Job drawing, mm, ordinate dimensions from the low corner. One solid piece. Round coordinates to 2 decimals unless told otherwise and drop trailing zeros. Write each loop counter-clockwise with the first axis right and the second up, starting at its lowest first coordinate (ties: lowest second). Pieces come first, ordered by that corner, then holes.
1) Flat gauge pins, fed straight in: pin 1 (3 mm diameter, centred on x = 4, y = 32, fed in from +Z) (1 decimal); pin 2 (4 mm diameter, centred on x = 19.5, y = 27, fed in from +Z) (1 decimal); pin 3 (2 mm diameter, centred on x = 18, y = 56.5, fed in from -Z) (1 decimal); pin 4 (2 mm diameter, centred on y = 33, z = 21, fed in from +X). Where does each tip first touch, or does it go through?
2) Pull direction X, two halves, no side cores. Call the marked faces 1 and 2: +X half, -X half, draft (parallel to the pull), parting line (faces both ways), or undercut.
3) Saw through at C-C (y = 38.5). Write the cut outline in (x, z) (1 decimal).
4) Saw through at A-A (x = 20.5). Write the cut outline in (y, z) (1 decimal).
5) Saw through at B-B (z = 27.5). Write the cut outline in (x, y) (1 decimal).
6) Wall check: probe 1 along X at (y, z) = (24, 31); probe 2 along Y at (x, z) = (19.75, 4.5) (1 decimal); probe 3 along Z at (x, y) = (21, 10) (1 decimal). Give the ranges that are in metal, low to high.
7) Saw through at D-D (x = 17.5). Write the cut outline in (y, z) (1 decimal).
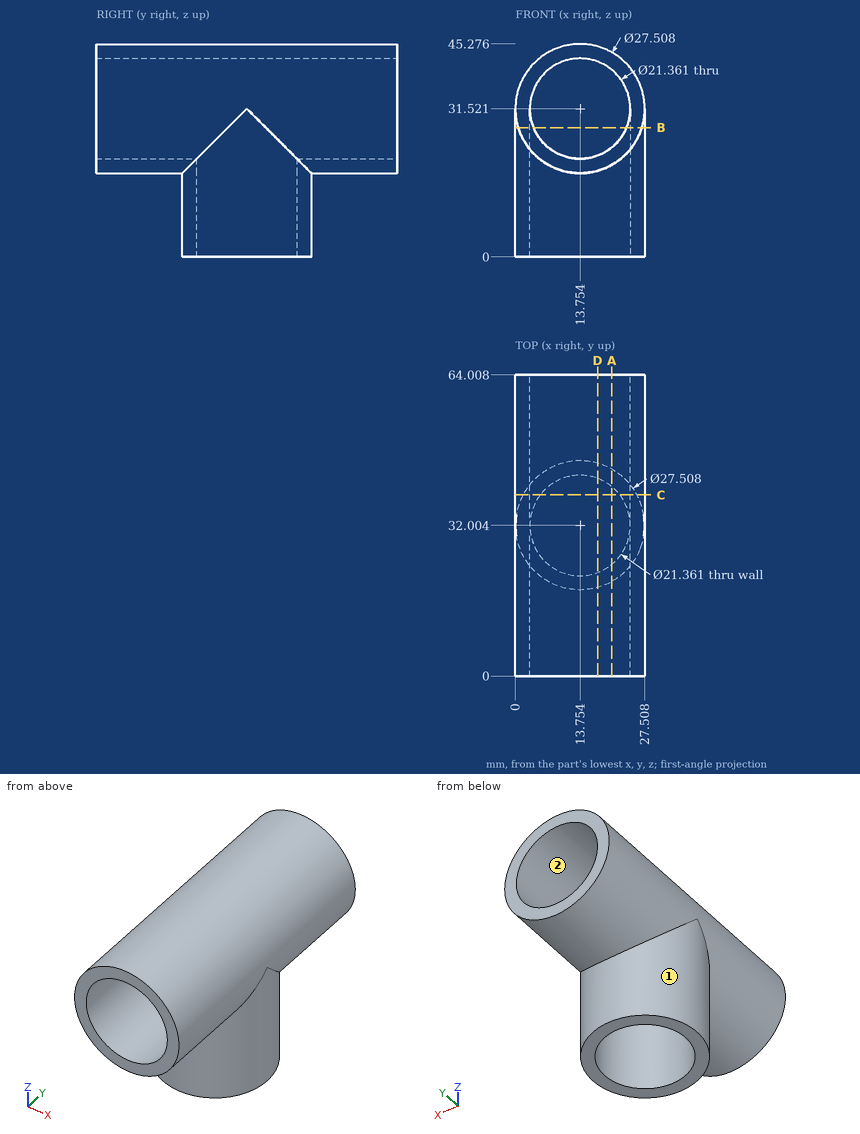
Evaluation:
1. pin 1: stops at z = 42.5
1. pin 2: stops at z = 44.8
1. pin 3: stops at z = 18.2
1. pin 4: stops at x = 27.51
2. face 1: parting line
2. face 2: undercut
3. outline: (1.6, 0) - (5.3, 0) - (5.3, 25) arc R10.7 cw (long way) to (22.2, 25) - (22.2, 0) - (25.9, 0) - (25.9, 25) arc R13.8 ccw (long way) to (1.6, 25) - close
4. outline: (0, 19.5) - (20, 19.5) - (20, 0) - (23.7, 0) - (23.7, 23.2) - (0, 23.2) - close; (0, 39.8) - (64, 39.8) - (64, 43.5) - (0, 43.5) - close; (40.3, 0) - (44, 0) - (44, 19.5) - (64, 19.5) - (64, 23.2) - (40.3, 23.2) - close
5. outline: (0.6, 0) - (3.9, 0) - (3.9, 28) arc R10.7 cw to (3.9, 36) - (3.9, 64) - (0.6, 64) - (0.6, 36) arc R13.8 ccw to (0.6, 28) - close; (23.6, 0) - (26.9, 0) - (26.9, 28) arc R13.8 ccw to (26.9, 36) - (26.9, 64) - (23.6, 64) - (23.6, 36) arc R10.7 cw to (23.6, 28) - close
6. probe 1: x = 0.01 to 3.09, 24.42 to 27.5
6. probe 2: y = 19.6 to 23.2, 40.8 to 44.4
6. probe 3: z = 19.8 to 23.7, 39.4 to 43.2
7. outline: (0, 18.3) - (18.8, 18.3) - (18.8, 0) - (22, 0) - (22, 21.5) - (0, 21.5) - close; (0, 41.5) - (64, 41.5) - (64, 44.8) - (0, 44.8) - close; (42, 0) - (45.2, 0) - (45.2, 18.3) - (64, 18.3) - (64, 21.5) - (42, 21.5) - close
